```python
from build123d import *

# Parameters (mm, degrees)
BOSS_EXTRUDE1_DEPTH = 3
BOSS_EXTRUDE2_DEPTH = 28
CUT_EXTRUDE1_DEPTH  = 30
CUT_EXTRUDE2_DEPTH  = 30
CUT_EXTRUDE3_REACH  = 55.204
CUT_EXTRUDE4_DEPTH  = 31
BOSS_EXTRUDE3_DEPTH = 15


with BuildPart() as part:
    # Sketch2 → Boss-Extrude1 (new body)
    with BuildSketch(Plane(origin=(0, 0, 0), x_dir=(1, 0, 0), z_dir=(0, 1, 0))):
        Polygon((-27.25, -8.405172527), (-27.25, -0.828427125), (-25.25, 0), (25.25, 0), (27.25, -0.828427125), (27.25, -8.405172527), (36.155887914, -12.094112086), (41.513455967, -6.736544033), (41.513455967, -3.489367432), (25.846737102, 3), (-25.846737102, 3), (-41.513455967, -3.489367432), (-41.513455967, -6.736544033), (-36.155887914, -12.094112086), align=None)
    extrude(amount=BOSS_EXTRUDE1_DEPTH)

    # Sketch3 → Boss-Extrude2 (add)
    with BuildSketch(Plane.XZ):
        Polygon((-41.513455967, 6.736544033), (-25.25, 0), (25.25, 0), (41.513455967, 6.736544033), (41.513455967, 3.489367432), (25.846737102, -3), (-25.846737102, -3), (-41.513455967, 3.489367432), align=None)
    extrude(amount=BOSS_EXTRUDE2_DEPTH)

    # Sketch4 → Cut-Extrude1 (cut, along a direction that is not the sketch's normal)
    with BuildSketch(Plane(origin=(-4.845827185, 0, -11.69886171), x_dir=(-0.9238795325112868, 0, 0.38268343236508967), z_dir=(-0.3826834323650896, 0, -0.9238795325112867))):
        Polygon((40.931396085, -14), (22.731221094, -28), (40.931396085, -28), align=None)
    extrude(amount=-CUT_EXTRUDE1_DEPTH, dir=(0, 0, -1), mode=Mode.SUBTRACT)

    # Sketch5 → Cut-Extrude2 (cut, along a direction that is not the sketch's normal)
    with BuildSketch(Plane(origin=(4.845827185, 0, -11.69886171), x_dir=(-0.923879532511309, 0, -0.3826834323650361), z_dir=(0.38268343236503605, 0, -0.9238795325113089))):
        Polygon((-40.931396085, -14), (-22.731221094, -28), (-40.931396085, -28), align=None)
    extrude(amount=-CUT_EXTRUDE2_DEPTH, dir=(0, 0, -1), mode=Mode.SUBTRACT)

    # Cut-Extrude3: up to this face of the body (flat: up to its plane)
    cut_extrude3_end = Plane(part.part.faces().sort_by_distance((0, -28, -1.498496392))[0])
    # Sketch6 → Cut-Extrude3 (cut, up to the picked face)
    with BuildSketch(Plane(origin=(0, 3, 0), x_dir=(1, 0, 0), z_dir=(0, 1, 0)), mode=Mode.PRIVATE) as cut_extrude3_sk1:
        Polygon((-39.809556561, -2.783589189), (-32.155887914, -10.437257836), (-36.155887914, -12.094112086), (-41.513455967, -6.736544033), (-41.513455967, -3.489367432), align=None)
    cut_extrude3_tool1 = split(extrude(cut_extrude3_sk1.sketch, amount=-CUT_EXTRUDE3_REACH, mode=Mode.PRIVATE), bisect_by=cut_extrude3_end, keep=Keep.BOTH, mode=Mode.PRIVATE)
    # Sketch6 → Cut-Extrude3 (cut, up to the picked face)
    with BuildSketch(Plane(origin=(0, 3, 0), x_dir=(1, 0, 0), z_dir=(0, 1, 0)), mode=Mode.PRIVATE) as cut_extrude3_sk2:
        Polygon((39.809556561, -2.783589189), (32.155887914, -10.437257836), (36.155887914, -12.094112086), (41.513455967, -6.736544033), (41.513455967, -3.489367432), align=None)
    cut_extrude3_tool2 = split(extrude(cut_extrude3_sk2.sketch, amount=-CUT_EXTRUDE3_REACH, mode=Mode.PRIVATE), bisect_by=cut_extrude3_end, keep=Keep.BOTH, mode=Mode.PRIVATE)
    add(cut_extrude3_tool1.solids().sort_by(Axis((-37.57796, 3, 7.679108), (0, -1, 0)))[0], mode=Mode.SUBTRACT)
    add(cut_extrude3_tool2.solids().sort_by(Axis((37.57796, 3, 7.679108), (0, -1, 0)))[0], mode=Mode.SUBTRACT)

    # Sketch7 → Cut-Extrude4 (cut)
    with BuildSketch(Plane(origin=(0, 3, 0), x_dir=(1, 0, 0), z_dir=(0, 1, 0))):
        Polygon((-25.25, 0), (-27.5, -0.931980515), (-27.5, -8.508725917), (27.5, -8.508725917), (27.5, -0.931980515), (25.25, 0), align=None)
    extrude(amount=-CUT_EXTRUDE4_DEPTH, mode=Mode.SUBTRACT)

    # Sketch8 → Boss-Extrude3 (add)
    with BuildSketch(Plane.XZ):
        Polygon((-32.155887914, 10.437257836), (-27.5, 8.508725917), (-27.5, 3.259123746), (-35.867917208, 6.725228542), align=None)
        Polygon((27.5, 3.259123746), (35.867917208, 6.725228542), (32.155887914, 10.437257836), (27.5, 8.508725917), align=None)
    extrude(amount=BOSS_EXTRUDE3_DEPTH)


solid = part.part
```
Part model, mm, in its own coordinate system. A direction names the side the tool comes from. Round coordinates to 2 decimals unless told otherwise and drop trailing zeros. Order: outer loops, then holes, each group sorted by start corner. A loop starts at its lowest first (then second) coordinate and runs counter-clockwise, first axis right, second up. Notation, with made-up numbers: M -19.5,-7 L 23.5,-7 A10 ccw 23.5,8 Z; hole C 74.5,-9 d11. An arc over 180 degrees is marked long. Answer in a Markdown table with one row per item. Add a question column.
Q1. Cut at D-D on z = -2. Give the cut face in (x, y).
Q2. Pin check, flat tips, straight feed: pin 1 (1.5 mm diameter, centred on y = -11.5, z = 6.5, fed in from -X); pin 2 (3 mm diameter, centred on x = -30.5, y = -1.5, fed in from +Z); pin 3 (5 mm diameter, centred on x = -26, y = -4.5, fed in from +Z). Stop position of each tip, or through.
Q3. Cut at A-A on y = -3.5. Give the cut face in (x, z).
Q4. Wall check: L1, parallel to X at y = -7.5, z = 4.5; L2, parallel to X at y = -10, z = 4; L3, parallel to Z at x = 8.5, y = -1.5. Give the ranges that are in metal, low to high. Write a range as from..to.
Q5. Cut at B-B on x = 21. Give the cut face in (y, z), and give its area (3 significant figures).
Q6. Cut at C-C on y = -23.5. Give the cut face in (x, z).
Q7. Mould opens along Z. For faces 1 (the face through (31.63, -7.4, 4.97)), 2 (the face through (-35.186, -7.494, 7.407)), 3 (the face through (-27.5, -6, 6)) say: +Z half, -Z half, draft (parallel to the pull), parting line (faces both ways), or undercut.
Q8. 3-axis set-ups, long thin cutter, end or side, ignore diameter. For faces 4 (the face through (0, -12, 0)), 5 (the face through (32.57, -22.4, 1.39)), 6 (the face through (32, 0, 4)): which of +Z, -Z, +X, -X, +Y, -Y reach the whole face in a straight line?
Established:
| question | item | result |
|---|---|---|
| 1 | outline | M -28.26,-25.99 L -25.85,-28 L 25.85,-28 L 28.26,-25.99 L 28.26,3 L -28.26,3 Z |
| 2 | pin 1 | stops at x = -35.87 |
| 2 | pin 2 | stops at z = 10.37 |
| 2 | pin 3 | stops at z = 8.92 |
| 3 | outline | M -39.81,2.78 L -25.85,-3 L 25.85,-3 L 39.81,2.78 L 37.51,5.08 L 25.25,0 L -25.25,0 L -37.51,5.08 Z; M -35.87,6.73 L -27.5,3.26 L -27.5,8.51 L -32.16,10.44 Z; M 27.5,3.26 L 35.87,6.73 L 32.16,10.44 L 27.5,8.51 Z |
| 4 | L1 | x = -38.09..-36.11, -30.5..-27.5, 27.5..30.5, 36.11..38.09 |
| 4 | L2 | x = -38.59..-34.91, -29.29..-27.5, 27.5..29.29, 34.91..38.59 |
| 4 | L3 | z = -3..0 |
| 5 | outline | M -28,-3 L 3,-3 L 3,0 L -28,0 Z |
| 5 | area | 93.0 mm2 |
| 6 | outline | M -31.25,-0.76 L -25.85,-3 L 25.85,-3 L 31.25,-0.76 L 31.25,2.49 L 25.25,0 L -25.25,0 L -31.25,2.49 Z |
| 7 | face 1 | undercut |
| 7 | face 2 | +Z half |
| 7 | face 3 | draft |
| 8 | face 4 | +Z, +Y, -Y |
| 8 | face 5 | +Z, -Z, +X, -Y |
| 8 | face 6 | -Y |
